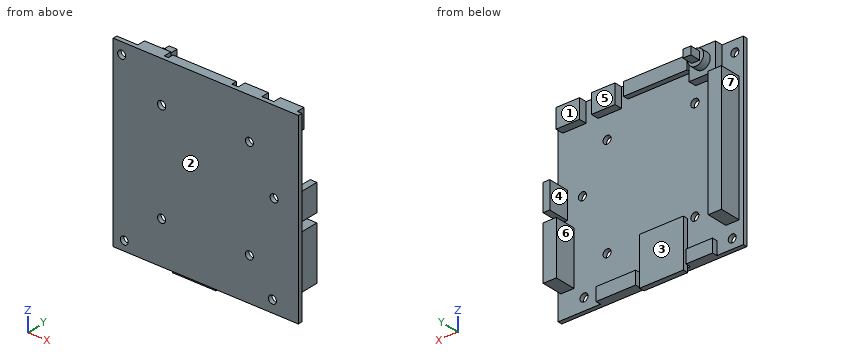
from build123d import *

# Parameters (mm, degrees)
SKETCH_1_W      = 70
SKETCH_1_H      = 70
SKETCH_1_R      = 1.55
SKETCH_1_R_2    = 1.5
EXTRUDE_1_DEPTH = 1.6
SKETCH_3_W      = 16.5
SKETCH_3_H      = 18.1
EXTRUDE_2_DEPTH = 2
SKETCH_5_W      = 8.9
SKETCH_5_H      = 7.3
EXTRUDE_3_DEPTH = 3
SKETCH_6_W      = 10
SKETCH_6_H      = 10
EXTRUDE_4_DEPTH = 3
SKETCH_7_R      = 3
EXTRUDE_5_DEPTH = 3
SKETCH_8_W      = 3
SKETCH_8_H      = 3
EXTRUDE_6_DEPTH = 4
SKETCH_9_W      = 24
SKETCH_9_H      = 5
SKETCH_9_W_2    = 10
SKETCH_9_W_3    = 15
EXTRUDE_7_DEPTH = 2
SKETCH_10_W     = 5
SKETCH_10_H     = 48.2
SKETCH_10_H_2   = 20.3
SKETCH_10_W_2   = 2.5
SKETCH_10_H_3   = 10.2
EXTRUDE_8_DEPTH = 8


with BuildPart() as part:
    # 草图1 → 凸台-拉伸1 (new body)
    with BuildSketch(Plane(origin=(0, 0, 0), x_dir=(1, 0, 0), z_dir=(0, 1, 0))):
        with Locations((16.69, 19.26)):
            Rectangle(SKETCH_1_W, SKETCH_1_H)
        with Locations(Location((0, 0, 0), (0, 0, 270))):
            Circle(SKETCH_1_R, mode=Mode.SUBTRACT)
        with Locations(Location((33.2, 0, 0), (0, 0, 270))):
            Circle(SKETCH_1_R_2, mode=Mode.SUBTRACT)
        with Locations(Location((0, 38.1, 0), (0, 0, 270))):
            Circle(SKETCH_1_R_2, mode=Mode.SUBTRACT)
        with Locations(Location((33.2, 38.1, 0), (0, 0, 270))):
            Circle(SKETCH_1_R_2, mode=Mode.SUBTRACT)
        with Locations(Location((-14.1, 50.64, 0), (0, 0, 270))):
            Circle(SKETCH_1_R_2, mode=Mode.SUBTRACT)
        with Locations(Location((41.9, 49.7, 0), (0, 0, 270))):
            Circle(SKETCH_1_R_2, mode=Mode.SUBTRACT)
        with Locations(Location((42.5, 15.5, 0), (0, 0, 270))):
            Circle(SKETCH_1_R_2, mode=Mode.SUBTRACT)
        with Locations(Location((-15.1, -11.4, 0), (0, 0, 270))):
            Circle(SKETCH_1_R_2, mode=Mode.SUBTRACT)
    extrude(amount=EXTRUDE_1_DEPTH)

    # 草图3 → 凸台-拉伸2 (add)
    with BuildSketch(Plane(origin=(0, 1.6, 0), x_dir=(1, 0, 0), z_dir=(0, 1, 0))):
        with Locations((10.95, 46.85)):
            Rectangle(SKETCH_3_W, SKETCH_3_H)
    extrude(amount=EXTRUDE_2_DEPTH)

    # 草图5 → 凸台-拉伸3 (add)
    with BuildSketch(Plane(origin=(0, 1.6, 0), x_dir=(1, 0, 0), z_dir=(0, 1, 0))):
        with Locations((45.54, -12.09)):
            Rectangle(SKETCH_5_W, SKETCH_5_H)
        with Locations((32.14, -12.09)):
            Rectangle(SKETCH_5_W, SKETCH_5_H)
    extrude(amount=EXTRUDE_3_DEPTH)

    # 草图6 → 凸台-拉伸4 (add)
    with BuildSketch(Plane(origin=(0, 1.6, 0), x_dir=(1, 0, 0), z_dir=(0, 1, 0))):
        with Locations((-5.31, -10.74)):
            Rectangle(SKETCH_6_W, SKETCH_6_H)
    extrude(amount=EXTRUDE_4_DEPTH)

    # 草图7 → 凸台-拉伸5 (add)
    with BuildSketch(Plane(origin=(0, 4.6, 0), x_dir=(1, 0, 0), z_dir=(0, 1, 0))):
        with Locations(Location((-5.31, -10.74, 0), (0, 0, 90))):
            Circle(SKETCH_7_R)
    extrude(amount=EXTRUDE_5_DEPTH)

    # 草图8 → 凸台-拉伸6 (add)
    with BuildSketch(Plane(origin=(0, 7.6, 0), x_dir=(1, 0, 0), z_dir=(0, 1, 0))):
        with Locations((-5.31, -10.74)):
            Rectangle(SKETCH_8_W, SKETCH_8_H)
    extrude(amount=EXTRUDE_6_DEPTH)

    # 草图9 → 凸台-拉伸7 (add)
    with BuildSketch(Plane(origin=(0, 1.6, 0), x_dir=(1, 0, 0), z_dir=(0, 1, 0))):
        with Locations((13.29, -13.24)):
            Rectangle(SKETCH_9_W, SKETCH_9_H)
        with Locations((-3.31, 51.76)):
            Rectangle(SKETCH_9_W_2, SKETCH_9_H)
        with Locations((28.19, 51.76)):
            Rectangle(SKETCH_9_W_3, SKETCH_9_H)
    extrude(amount=EXTRUDE_7_DEPTH)

    # 草图10 → 凸台-拉伸8 (add)
    with BuildSketch(Plane(origin=(0, 1.6, 0), x_dir=(1, 0, 0), z_dir=(0, 1, 0))):
        with Locations((-14.21, 21.26)):
            Rectangle(SKETCH_10_W, SKETCH_10_H)
        with Locations((48.19, 35.11)):
            Rectangle(SKETCH_10_W, SKETCH_10_H_2)
        with Locations((49.44, 16.46)):
            Rectangle(SKETCH_10_W_2, SKETCH_10_H_3)
    extrude(amount=EXTRUDE_8_DEPTH)


solid = part.part
The model under review builds one solid part; all positions refer to its coordinate system, in mm. Face numbers are marked on the shaded views. A direction names the side the tool comes from. Round coordinates to 2 decimals unless told otherwise and drop trailing zeros. Write each loop counter-clockwise with the first axis right and the second up, starting at its lowest first coordinate (ties: lowest second). Pieces come first, ordered by that corner, then holes. Notation, with made-up numbers: M -8.75,14.25 L 40.25,14.25 A12 cw 40.25,21.25 Z; hole C -7,44.25 d5. An arc over 180 degrees is marked long. Use a Markdown table: item, result. Add a question column.
Q1. Insertion check: pin 1 (2 mm diameter, centred on y = 2.5, z = -44.5, fed in from -X); pin 2 (6 mm diameter, centred on y = 7.5, z = -42, fed in from -X); pin 3 (3.5 mm diameter, centred on y = 9, z = 11, fed in from +X); pin 4 (0.6 mm diameter, centred on y = 2, z = 12.5, fed in from -X). Each pin has a flat end and moves straight along its axis. Give the tip position at first contact, or say it passes through.
Q2. Machinability: for the marked faces 1, 2, 3 and 4, which of the approach directions +Z, -Z, +X, -X, +Y, -Y give a long, thin tool a straight path to every point of the face, cutting with its end or side? Answer none if there is none.
Q3. The part is to be moulded in two halves that separate along X. For the marked faces 5, 6 and 7, say which applies: pulls with the +X half, pulls with the -X half, needs draft (parallel to the pull), parting line crosses it, or undercut.
Q4. We need section A-A, the plane x = 33.2. State the section outline as (y, z) points, plus the area to 3 significant figures.
Q5. We need section D-D, the plane x = 16.5. State the section outline as (y, z) points, plus the area to 3 significant figures.
Q6. We need section C-C, the plane z = -4.5. State the section outline as (x, y) points.
Q7. To check wall thickness, follow line 1 (X direction, y = 1.1, z = -38.1); line 2 (X direction, y = 0.35, z = 11.4); line 3 (Z direction, x = -3.5, y = 2.5). State the ranges of each line that lie inside material, in increasing order.
Q8. We need section B-B, the plane y = 6.25. State the section outline as (x, z) points, plus the area to 3 significant figures.
Findings below:
| question | item | result |
|---|---|---|
| 1 | pin 1 | stops at x = -18.31 |
| 1 | pin 2 | stops at x = -16.71 |
| 1 | pin 3 | stops at x = -2.31 |
| 1 | pin 4 | stops at x = -10.31 |
| 2 | face 1 | +Z, +X, +Y |
| 2 | face 2 | +Z, -Z, +X, -X, -Y |
| 2 | face 3 | +Z, -Z, +Y |
| 2 | face 4 | +Y |
| 3 | face 5 | needs draft |
| 3 | face 6 | undercut |
| 3 | face 7 | pulls with the -X half |
| 4 | outline | M 0,-54.26 L 3.6,-54.26 L 3.6,-49.26 L 1.6,-49.26 L 1.6,-39.6 L 0,-39.6 Z; M 0,-36.6 L 1.6,-36.6 L 1.6,-1.5 L 0,-1.5 Z; M 0,1.5 L 1.6,1.5 L 1.6,8.44 L 4.6,8.44 L 4.6,15.74 L 0,15.74 Z |
| 4 | area | 134 mm² |
| 5 | outline | M 0,-54.26 L 1.6,-54.26 L 1.6,-55.9 L 3.6,-55.9 L 3.6,-37.8 L 1.6,-37.8 L 1.6,10.74 L 3.6,10.74 L 3.6,15.74 L 0,15.74 Z |
| 5 | area | 158 mm² |
| 6 | outline | M -18.31,0 L 51.69,0 L 51.69,1.6 L -11.71,1.6 L -11.71,9.6 L -16.71,9.6 L -16.71,1.6 L -18.31,1.6 Z |
| 7 | line 1 | x = -18.31 to -1.5, 1.5 to 31.7, 34.7 to 51.69 |
| 7 | line 2 | x = -18.31 to -16.6, -13.6 to 51.69 |
| 7 | line 3 | z = -54.26 to -49.26, 5.74 to 15.74 |
| 8 | outline | M -16.71,-45.36 L -11.71,-45.36 L -11.71,2.84 L -16.71,2.84 Z; C -5.31,10.74 d6; M 45.69,-45.26 L 50.69,-45.26 L 50.69,-24.96 L 45.69,-24.96 Z; M 48.19,-21.56 L 50.69,-21.56 L 50.69,-11.36 L 48.19,-11.36 Z |
| 8 | area | 396 mm² |
